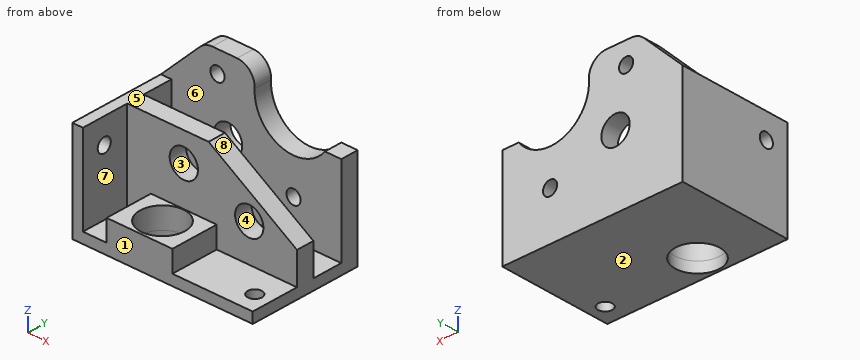
```python
from build123d import *

# Parameters (mm, degrees)
F0_W      = 51
F0_H      = 32
F0_R      = 2
F1_DEPTH  = 3
F3_DEPTH  = 25
F2_W      = 18.6
F2_H      = 13.5
F2_R      = 6.3
F4_DEPTH  = 6
F5_DEPTH  = 3
F6_SIZE2  = 16
F6_SIZE   = 25
F7_R      = 4
F8_DEPTH  = 18.501
F7_R_2    = 2
F9_DEPTH  = 18.501
F10_DEPTH = 5
F12_DEPTH = 12.5
F13_R     = 2
F14_DEPTH = 5
F15_SIZE  = 12.5
F16_R     = 5
F17_R     = 2
F18_DEPTH = 3


with BuildPart() as f1:
    # F0 (on Top) → F1 (new body)
    with BuildSketch(Plane.XY):
        Rectangle(F0_W, F0_H)
        with Locations((21, -10.5)):
            Circle(F0_R, mode=Mode.SUBTRACT)
    extrude(amount=F1_DEPTH)

    # F2 (on face) → F3 (join)
    with BuildSketch(Plane.XY.offset(3)):
        Polygon((-22.5, 2.5), (-22.5, 11), (25.5, 11), (25.5, 16), (-25.5, 16), (-25.5, -16), (-22.5, -16), (-22.5, -2.5), (-15.8, -2.5), (2.8, -2.5), (25.5, -2.5), (25.5, 2.5), align=None)
    extrude(amount=F3_DEPTH)

    # F2 (on face) → F4 (join)
    with BuildSketch(Plane.XY.offset(3)):
        with Locations((-6.5, -9.25)):
            Rectangle(F2_W, F2_H)
        with Locations((-6.5, -9)):
            Circle(F2_R, mode=Mode.SUBTRACT)
    extrude(amount=F4_DEPTH)

    # F5 (cut, through all): a face of the model
    f5_faces = [f1.faces().sort_by_distance(p)[0] for p in [
        (-6.5, -9, 3),
    ]]
    extrude(f5_faces, amount=-F5_DEPTH, mode=Mode.SUBTRACT)

    # F6
    f6_edges = [f1.edges().sort_by_distance(p)[0] for p in [
        (25.5, 0, 28),
    ]]
    f6_side = f1.faces().sort_by_distance((-23.10208, 6.75, 28))[0]
    chamfer(f6_edges, length=F6_SIZE, length2=F6_SIZE2, reference=f6_side)

    # F7 (on face) → F8 (cut, through all)
    with BuildSketch(Plane.XZ.offset(2.5)):
        with Locations((-6.5, 20)):
            Circle(F7_R)
    extrude(amount=-F8_DEPTH, mode=Mode.SUBTRACT)

    # F7 (on face) → F9 (cut, through all)
    with BuildSketch(Plane.XZ.offset(2.5)):
        with Locations((12, 13.5)):
            Circle(F7_R_2)
    extrude(amount=-F9_DEPTH, mode=Mode.SUBTRACT)

    # F7 (on face) → F10 (cut, through all)
    with BuildSketch(Plane.XZ.offset(2.5)):
        with Locations((12, 13.5)):
            Circle(F7_R)
        with Locations((12, 13.5)):
            Circle(F7_R_2, mode=Mode.SUBTRACT)
    extrude(amount=-F10_DEPTH, mode=Mode.SUBTRACT)

    # F11 (on face) → F12 (join)
    with BuildSketch(Plane.XY.offset(28)):
        Polygon((-25.5, 11), (-22.5, 11), (25.5, 11), (25.5, 16), (-25.5, 16), align=None)
    extrude(amount=F12_DEPTH)

    # F13 (on face) → F14 (cut, through all)
    with BuildSketch(Plane(origin=(0, 16, 0), x_dir=(-1, 0, 0), z_dir=(0, 1, 0))):
        with Locations((9.5, 34.5)):
            Circle(F13_R)
        with BuildLine():
            Line((-25.5, 28), (-20.8741196746, 28))
            ThreePointArc((-20.8741196746, 28), (-5.7476140898, 25.4497143454), (-2.7804555427, 40.5))
            Line((-2.7804555427, 40.5), (-25.5, 40.5))
            Line((-25.5, 40.5), (-25.5, 28))
        make_face()
    extrude(amount=-F14_DEPTH, mode=Mode.SUBTRACT)

    # F15
    f15_edges = [f1.edges().sort_by_distance(p)[0] for p in [
        (-25.5, 13.5, 40.5),
    ]]
    chamfer(f15_edges, length=F15_SIZE)

    # F16
    f16_edges = [f1.edges().sort_by_distance(p)[0] for p in [
        (2.780456, 13.5, 40.5),
        (-13, 13.5, 40.5),
    ]]
    fillet(f16_edges, radius=F16_R)

    # F17 (on face) → F18 (cut, through all)
    with BuildSketch(Plane(origin=(-25.5, 0, 0), x_dir=(0, -1, 0), z_dir=(-1, 0, 0))):
        with Locations((9.5, 21)):
            Circle(F17_R)
    extrude(amount=-F18_DEPTH, mode=Mode.SUBTRACT)


solid = f1.part
```
For this review, take the finished solid that the model builds, in its own axes (mm). Face numbers are marked on the shaded views. A direction names the side the tool comes from. Coordinates: 2 decimals unless noted, no trailing zeros. Loops run counter-clockwise (first coordinate to the right, second up) from the corner with the lowest first, then second, coordinate; pieces in that order, holes last. Notation, with made-up numbers: (84.25, -23) - (143.25, -23) arc R14 cw to (143.25, 1) - close; hole circle Ø7 at (-36.5, -0.75). An arc over 180 degrees is marked (long way). Use one line per item in the form item = value. Start each with the question number.
1) Take a section at D-D (z = 34.5). State the section outline as (x, y) points, plus the area to 3 significant figures.
2) For the marked faces 4, 5, 6, 7 and 8, list the 3-axis set-ups (+Z, -Z, +X, -X, +Y, -Y) from which the entire face can be reached by the end or side of a thin tool; tool diameter is ignored.
3) Draft analysis for pull direction Z (two halves, no side actions). For the marked faces 1, 2 and 3, state which applies: released by +Z, released by -Z, zero draft, split by the parting line, or undercut.
4) Take a section at B-B (z = 5.5). State the section outline as (x, y) points, plus the area to 3 significant figures.
5) For pin 1 (2 mm diameter, centred on x = -18, y = -11.5, fed in from +Z); pin 2 (3.5 mm diameter, centred on x = 12, z = 13.5, fed in from -Y); pin 3 (13 mm diameter, centred on x = 12, z = 13.5, fed in from +Y); pin 4 (5 mm diameter, centred on y = -12, z = 6, fed in from +X), all flat-tipped, find the tip position at first contact; note any pin that passes through.
6) Take a section at C-C (y = -6). State the section outline as (x, z) points, plus the area to 3 significant figures.
7) To check wall thickness, follow probe 1 along Y at (x, z) = (-10.5, 27); probe 2 along Y at (x, z) = (21, 1); probe 3 along Z at (x, y) = (-9.5, 13.75). State the ranges of each line that lie inside material, in increasing order. Write a range as from..to.
8) Take a section at A-A (x = -6.5). State the section outline as (y, z) points.
From the geometry:
q1.outline = (-19, 11) - (-11.5, 11) - (-11.5, 16) - (-19, 16) - close; (-7.5, 11) - (1, 11) - (1, 16) - (-7.5, 16) - close
q1.area = 80.0 mm2
q2.face_4 = -Y
q2.face_5 = +Z, +X, -X, -Y
q2.face_6 = +Z, +X
q2.face_7 = +Z, -Y
q2.face_8 = +Z, +X, -Y
q3.face_1 = zero draft
q3.face_2 = released by -Z
q3.face_3 = undercut
q4.outline = (-25.5, -16) - (-22.5, -16) - (-22.5, -2.5) - (-15.8, -2.5) - (-15.8, -16) - (2.8, -16) - (2.8, -2.5) - (25.5, -2.5) - (25.5, 2.5) - (-22.5, 2.5) - (-22.5, 11) - (25.5, 11) - (25.5, 16) - (-25.5, 16) - close; hole circle Ø12.6 at (-6.5, -9)
q4.area = 702 mm2
q5.pin_1 = 3
q5.pin_2 = through
q5.pin_3 = 16
q5.pin_4 = 2.8
q6.outline = (-25.5, 0) - (-12.04, 0) - (-12.04, 9) - (-15.8, 9) - (-15.8, 3) - (-22.5, 3) - (-22.5, 28) - (-25.5, 28) - close; (-0.96, 0) - (25.5, 0) - (25.5, 3) - (2.8, 3) - (2.8, 9) - (-0.96, 9) - close
q6.area = 240 mm2
q7.probe_1 = -2.5..2.5, 11..16
q7.probe_2 = -16..-12.5, -8.5..16
q7.probe_3 = 0..17.35, 22.65..32.5, 36.5..40.5
q8.outline = (-16, 0) - (-15.3, 0) - (-15.3, 9) - (-16, 9) - close; (-2.7, 0) - (16, 0) - (16, 16) - (11, 16) - (11, 3) - (2.5, 3) - (2.5, 16) - (-2.5, 16) - (-2.5, 9) - (-2.7, 9) - close; (-2.5, 24) - (2.5, 24) - (2.5, 28) - (-2.5, 28) - close; (11, 24) - (16, 24) - (16, 40.5) - (11, 40.5) - close
